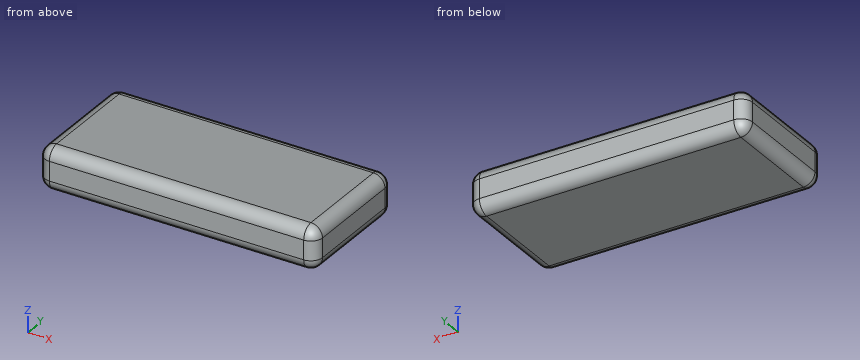
```python
from build123d import *

# Parameters (mm, degrees)
F0_W     = 45.72
F0_H     = 6.985
F1_DEPTH = 10.16
F2_R     = 1.905
F6_ANGLE = 180
F3_W     = 12.446
F3_H     = 2.286
F7_DEPTH = 5.207
F4_W     = 7.62
F4_H     = 1.778
F8_DEPTH = 7.8105


# Not quite as in the source:
# - a length typed as a fraction of an inch, garbled in the dataset ("3 / 203.2 mm" for 3/8 in), is restored


with BuildPart() as f1:
    # F0 (on Front) → F1 (new body)
    with BuildSketch(Plane.XZ):
        Rectangle(F0_W, F0_H)
    extrude(amount=-F1_DEPTH)

    # F2
    f2_edges = [f1.edges().sort_by_distance(p)[0] for p in [
        (0, 10.16, 3.4925),
        (22.86, 5.08, 3.4925),
        (22.86, 10.16, 0),
        (22.86, 5.08, -3.4925),
        (-22.86, 10.16, 0),
        (-22.86, 5.08, -3.4925),
        (-22.86, 5.08, 3.4925),
        (0, 10.16, -3.4925),
    ]]
    fillet(f2_edges, radius=F2_R)

    # F5 (on face) → F6 (revolve, cut)
    with BuildSketch(Plane.XZ):
        Polygon((13.97, -1.5621), (18.542, -0.5461), (18.542, 0.5969), (20.32, 0.5969), (20.32, 2.3749), (12.446, 2.3749), (12.446, -3.0861), (13.97, -3.0861), align=None)
    revolve(axis=Axis((12.446, 0, -0.3556), (0, 0, 1)), revolution_arc=F6_ANGLE, mode=Mode.SUBTRACT)

    # F3 (on face) → F7 (cut)
    with BuildSketch(Plane.XZ):
        with Locations((-14.097, 0)):
            Rectangle(F3_W, F3_H)
    extrude(amount=-F7_DEPTH, mode=Mode.SUBTRACT)

    # F4 (on face) → F8 (cut)
    with BuildSketch(Plane.XZ):
        with Locations((-1.27, 0)):
            Rectangle(F4_W, F4_H)
    extrude(amount=-F8_DEPTH, mode=Mode.SUBTRACT)

    # F9: F1 across face


with BuildPart() as f1_1:
    add(f1.part)
    add(f1.part.mirror(Plane(origin=(-1.1723055417, 0, -0.108173269), x_dir=(1, 0, 0), z_dir=(0, -1, 0))))


solid = f1_1.part
```
Part model, mm, in its own coordinate system. Coordinates: 2 decimals unless noted, no trailing zeros. Write each loop counter-clockwise with the first axis right and the second up, starting at its lowest first coordinate (ties: lowest second). Pieces come first, ordered by that corner, then holes.
Item 1: Slice it at C-C (z = -2.5). Write the cut outline in (x, y) (3 decimals).
Item 2: Slice it at B-B (y = -7.25). Write the cut outline in (x, z) (1 decimal), and give its area (3 significant figures).
Item 3: Probe line 1 (Z direction, x = -19, y = -1); line 2 (X direction, y = 6.5, z = -0.25); line 3 (Z direction, x = -5, y = 7). List the from-to ranges inside material, lowest first.
Item 4: Slice it at D-D (y = -3.5). Count the separate pieces of the cut face and the enclosed holes in it, and give its area (3 significant figures).
Item 5: Slice it at A-A (x = 3). Write the cut outline in (y, z) (1 decimal).
Results found:
1. outline: (-22.627, -8.255) arc R1.672 ccw to (-20.955, -9.927) - (20.955, -9.927) arc R1.672 ccw to (22.627, -8.255) - (22.627, 8.255) arc R1.672 ccw to (20.955, 9.927) - (-20.955, 9.927) arc R1.672 ccw to (-22.627, 8.255) - close; hole circle Ø3.048 at (12.446, 0)
2. outline: (-22.9, -1.6) arc R1.9 ccw to (-21, -3.5) - (21, -3.5) arc R1.9 ccw to (22.9, -1.6) - (22.9, 1.6) arc R1.9 ccw to (21, 3.5) - (-21, 3.5) arc R1.9 ccw to (-22.9, 1.6) - close; hole (-5.1, -0.9) - (2.5, -0.9) - (2.5, 0.9) - (-5.1, 0.9) - close; hole (9.4, 0.6) - (15.5, 0.6) - (15.5, 2.4) - (9.4, 2.4) - close
2. area: 292 mm2
3. line 1: z = -3.49 to -1.14, 1.14 to 3.49
3. line 2: x = -22.86 to -5.08, 2.54 to 22.86
3. line 3: z = -3.49 to -0.89, 0.89 to 3.49
4. separate pieces: 1
4. enclosed holes: 3
4. area: 234 mm2
5. outline: (-10.2, -1.6) arc R1.9 ccw to (-8.3, -3.5) - (8.3, -3.5) arc R1.9 ccw to (10.2, -1.6) - (10.2, 1.6) arc R1.9 ccw to (8.3, 3.5) - (-8.3, 3.5) arc R1.9 ccw to (-10.2, 1.6) - close
